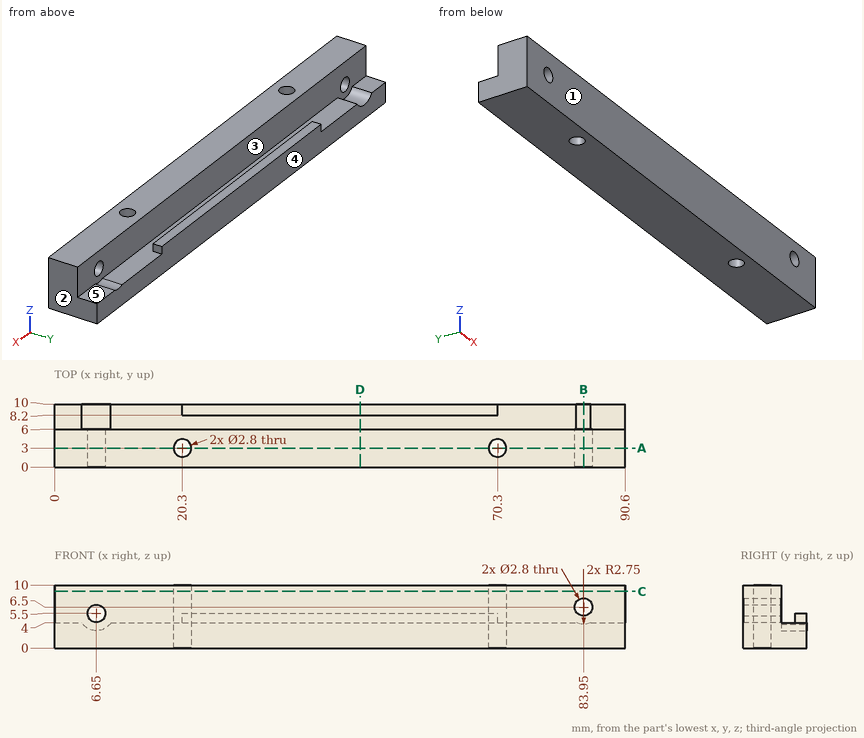
Answer from the drawing. Dimensions are ordinates in mm from the lowest x, y and z of the part. A direction names the side the tool comes from. Round coordinates to 2 decimals unless told otherwise and drop trailing zeros. Order: outer loops, then holes, each group sorted by start corner. A loop starts at its lowest first (then second) coordinate and runs counter-clockwise, first axis right, second up. Notation, with made-up numbers: (-29, 63.25) - (7, 63.25) arc R19 ccw to (7, 97.25) - close; hole circle Ø7 at (28.5, 2.5). An arc over 180 degrees is marked (long way). Put each result on its own line as item: value. Start each with the question number.
(1) Find section B-B (x = 83.95). Give the vertices of the cut face in (y, z).
(2) Straight lines are drawn through the part: probe 1 along Z at (x, y) = (83.95, 3.85); probe 2 along Z at (x, y) = (6.65, 3.65); probe 3 along X at (y, z) = (3.75, 7). For each, find the intervals that lie inside material, in ascending order. Write a range as from..to.
(3) Find section A-A (y = 3). Give the vertices of the cut face in (x, z), plus the area to 3 significant figures.
(4) Find section C-C (z = 9). Give the vertices of the cut face in (x, y), plus the area to 3 significant figures.
(5) Given P1, Ø2, axis at x = 42, y = 9, coming from the +Z side; P2, Ø2, axis at x = 6.65, z = 5.5, coming from the -Y side (3 decimals); P3, Ø3, axis at x = 1, y = 8.5, coming from the +Z side; P4, Ø5, axis at x = 17, z = 7, coming from the +Y side, each flat-ended and moving along its own axis, determine where each tip first touches the part or whether it passes through.
(6) Find section D-D (x = 48.5). Give the vertices of the cut face in (y, z).
(7) Determine the mould class of the marked faces 1, 2 and 3 for opening direction Y: released by +Y, released by -Y, zero draft, split by the parting line, or undercut.
(8) For the marked faces 4 and 5, determine the directions among +Z, -Z, +X, -X, +Y, -Y from which every point of the face is accessible in a straight line to the end or side of a thin tool.
Reply:
1. outline: (0, 0) - (10, 0) - (10, 3.75) - (6, 3.75) - (6, 5.1) - (0, 5.1) - close; (0, 7.9) - (6, 7.9) - (6, 10) - (0, 10) - close
2. probe 1: 0..5.1, 7.9..10
2. probe 2: 0..4.1, 6.9..10
2. probe 3: 0..19.12, 21.48..69.12, 71.48..82.64, 85.26..90.6
3. outline: (0, 0) - (18.9, 0) - (18.9, 10) - (0, 10) - close; (21.7, 0) - (68.9, 0) - (68.9, 10) - (21.7, 10) - close; (71.7, 0) - (90.6, 0) - (90.6, 10) - (71.7, 10) - close; hole circle Ø2.8 at (6.65, 5.5); hole circle Ø2.8 at (83.95, 6.5)
3. area: 838 mm^2
4. outline: (0, 0) - (90.6, 0) - (90.6, 6) - (0, 6) - close; hole circle Ø2.8 at (20.3, 3); hole circle Ø2.8 at (70.3, 3)
4. area: 531 mm^2
5. P1: z = 5.5
5. P2: through
5. P3: z = 4
5. P4: y = 6
6. outline: (0, 0) - (10, 0) - (10, 5.5) - (8.2, 5.5) - (8.2, 4) - (6, 4) - (6, 10) - (0, 10) - close
7. face 1: released by -Y
7. face 2: zero draft
7. face 3: undercut
8. face 4: +Z, -Z, +X, -X, +Y
8. face 5: +Z, +X, +Y
